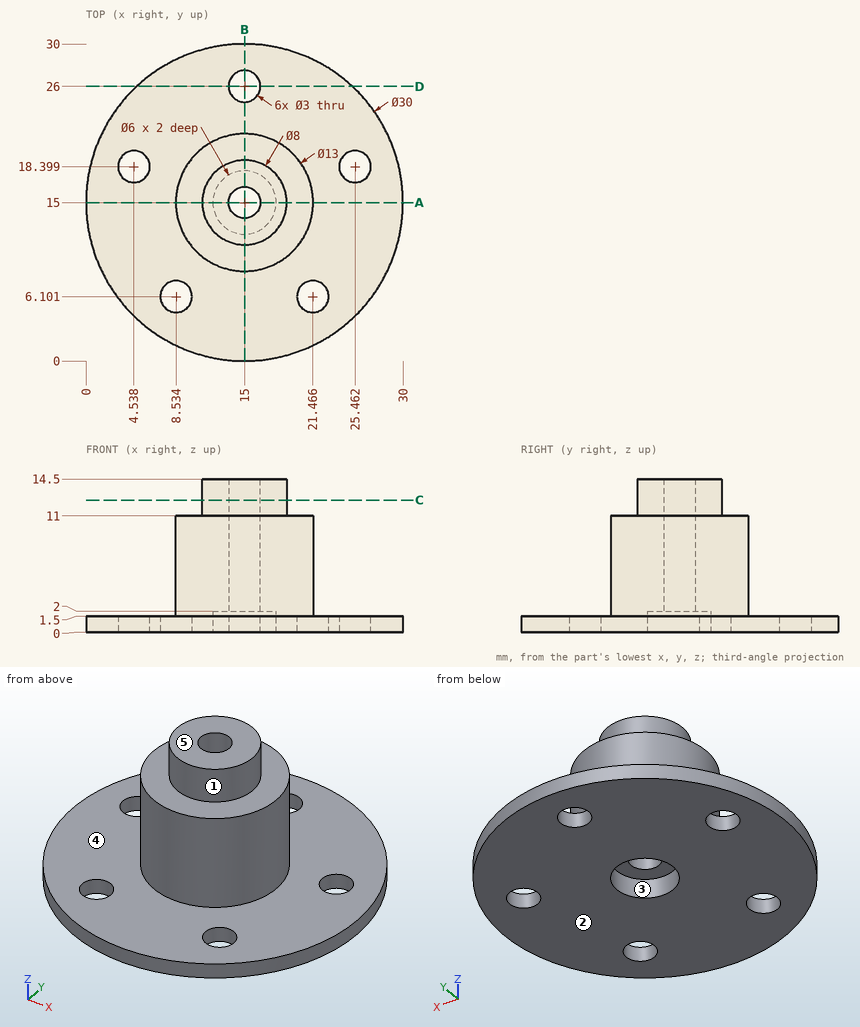
Geometry: see drawing. Coordinates: mm, zero at the bounding-box minimum. A direction names the side the tool comes from. Coordinates: 2 decimals unless noted, no trailing zeros. Loops run counter-clockwise (first coordinate to the right, second up) from the corner with the lowest first, then second, coordinate; pieces in that order, holes last.
(1) Set-up query: the marked faces 4 and 5. Return all of +Z, -Z, +X, -X, +Y, -Y with unobstructed straight access to the full face (end or side cutting, diameter ignored); none if empty.
(2) Section C-C on z = 12.5. Return the cut outline in (x, y).
(3) Section D-D on y = 26. Return the cut outline in (x, z), then the cut area to 3 significant figures.
(4) Material intervals for probe 1 along Y at (x, z) = (15, 0.75); probe 2 along Y at (x, z) = (15, 4.5); probe 3 along Z at (x, y) = (25, 10), sorted ascending.
(5) Section A-A on y = 15. Return the cut outline in (x, z).
(6) Section B-B on x = 15. Return the cut outline in (y, z).
(7) First-contact query: pin 1 Ø3.5 at (x, y) = (8.53, 6.1) entering from +Z; pin 2 Ø8 at (x, z) = (8.5, 10) entering from +Y; pin 3 Ø1.5 at (y, z) = (10.5, 10.5) entering from +X; pin 4 Ø1.8 at (x, y) = (21.47, 6.1) entering from +Z. Flat tips, straight axial feed; report the tip coordinate or a pass-through.
(8) Pull-direction query (Y, two-part tool) for the marked faces 1, 2 and 3; classes: released by +Y, released by -Y, zero draft, split by the parting line, or undercut.
Data:
1. face 4: +Z
1. face 5: +Z, +X, -X, +Y, -Y
2. outline: circle Ø8 at (15, 15); hole circle Ø3 at (15, 15)
3. outline: (4.8, 0) - (13.5, 0) - (13.5, 1.5) - (4.8, 1.5) - close; (16.5, 0) - (25.2, 0) - (25.2, 1.5) - (16.5, 1.5) - close
3. area: 26.1 mm2
4. probe 1: y = 0 to 12, 18 to 24.5, 27.5 to 30
4. probe 2: y = 8.5 to 13.5, 16.5 to 21.5
4. probe 3: z = 0 to 1.5
5. outline: (0, 0) - (12, 0) - (12, 2) - (13.5, 2) - (13.5, 14.5) - (11, 14.5) - (11, 11) - (8.5, 11) - (8.5, 1.5) - (0, 1.5) - close; (16.5, 2) - (18, 2) - (18, 0) - (30, 0) - (30, 1.5) - (21.5, 1.5) - (21.5, 11) - (19, 11) - (19, 14.5) - (16.5, 14.5) - close
6. outline: (0, 0) - (12, 0) - (12, 2) - (13.5, 2) - (13.5, 14.5) - (11, 14.5) - (11, 11) - (8.5, 11) - (8.5, 1.5) - (0, 1.5) - close; (16.5, 2) - (18, 2) - (18, 0) - (24.5, 0) - (24.5, 1.5) - (21.5, 1.5) - (21.5, 11) - (19, 11) - (19, 14.5) - (16.5, 14.5) - close; (27.5, 0) - (30, 0) - (30, 1.5) - (27.5, 1.5) - close
7. pin 1: stops at z = 1.5
7. pin 2: stops at y = 21
7. pin 3: stops at x = 20.31
7. pin 4: passes through
8. face 1: split by the parting line
8. face 2: zero draft
8. face 3: undercut
